Work out the finished part from the listing and answer in its coordinate system (mm). A direction names the side the tool comes from. Round coordinates to 2 decimals unless told otherwise and drop trailing zeros. Order: outer loops, then holes, each group sorted by start corner. A loop starts at its lowest first (then second) coordinate and runs counter-clockwise, first axis right, second up. Notation, with made-up numbers: M 41.25,2 L 50.25,2 A38 ccw 50.25,41 Z; hole C 85,66 d6. An arc over 180 degrees is marked long. Return JSON: item names as keys, results as strings.
from build123d import *

# Parameters (mm, degrees)
F0_R     = 19.7104
F0_R_2   = 17.1704
F1_DEPTH = 54.6227
F3_DEPTH = 19.7114
F5_DEPTH = 25.4


with BuildPart() as f1:
    # F0 (on Front) → F1 (new body, symmetric)
    with BuildSketch(Plane.XZ):
        Circle(F0_R)
        Circle(F0_R_2, mode=Mode.SUBTRACT)
    extrude(amount=F1_DEPTH, both=True)

    # F2 (on Top) → F3 (cut, through all)
    with BuildSketch(Plane.XY):
        with BuildLine():
            ThreePointArc((0, 52.7177), (-0.898026, 52.345726), (-1.27, 51.4477))
            Line((-1.27, 51.4477), (-1.27, -43.4721))
            ThreePointArc((-1.27, -43.4721), (-0.898026, -44.370126), (0, -44.7421))
            ThreePointArc((0, -44.7421), (0.898026, -44.370126), (1.27, -43.4721))
            Line((1.27, -43.4721), (1.27, 51.4477))
            ThreePointArc((1.27, 51.4477), (0.898026, 52.345726), (0, 52.7177))
        make_face()
    extrude(amount=F3_DEPTH, mode=Mode.SUBTRACT)

    # F4 (on Right) → F5 (cut, symmetric)
    with BuildSketch(Plane.YZ):
        with BuildLine():
            Line((-54.6227, 19.7104), (-54.6227, -19.7104))
            ThreePointArc((-54.6227, -19.7104), (-48.2727, 0), (-54.6227, 19.7104))
        make_face()
    extrude(amount=F5_DEPTH, both=True, mode=Mode.SUBTRACT)


solid = f1.part
Item 1: Which of the six approach directions +Z, -Z, +X, -X, +Y, -Y give full straight-line access (tool end or side, diameter ignored) to faces 4 (the cylindrical face through (14.692, -49.587, -9.331)), 5 (the flat face through (1.27, 3, 18))?
Output:
{"face 4": "+X, -X, -Y", "face 5": "+Z"}
Item 2: The mould has two halves that part along X. Classify faces 1 (the cylindrical face through (16.378, 1.582, 5.158)), 2 (the cylindrical face through (-19.69, -0.77, 0.87)), 3 (the flat face through (1, 54.623, 18)): pulls with the +X half, pulls with the -X half, needs draft (parallel to the pull), parting line crosses it, or undercut.
Output:
{"face 1": "undercut", "face 2": "parting line crosses it", "face 3": "needs draft"}
Item 3: Each of these flat-tipped pins is pushed along its axis until it touches: pin 1 (2 mm diameter, centred on y = 40.5, z = 12, fed in from -X); pin 2 (10 mm diameter, centred on y = -21.5, z = -1, fed in from +X); pin 3 (2 mm diameter, centred on x = -11.5, y = -2.5, fed in from -Z); pin 4 (1 mm diameter, centred on x = 15.5, y = 9.5, fed in from -Z). Where does it stop, or does it pass through?
Output:
{"pin 1": "stops at x = -16.36", "pin 2": "stops at x = 19.71", "pin 3": "stops at z = -16.68", "pin 4": "stops at z = -12.79"}
Item 4: Find section C-C (y = -12). Determine the outline of the cut face in (x, z), plus the area to 3 significant figures.
Output:
{"outline": "M -1.27,17.12 L -1.27,19.67 A19.71 ccw long 1.27,19.67 L 1.27,17.12 A17.17 cw long Z", "area": "288 mm^2"}
Item 5: Find section A-A (z = 0). Determine the outline of the cut face in (x, y).
Output:
{"outline": "M -19.71,-48.27 L -17.17,-48.27 L -17.17,54.62 L -19.71,54.62 Z; M 17.17,-48.27 L 19.71,-48.27 L 19.71,54.62 L 17.17,54.62 Z"}
Item 6: Find section B-B (x = -12.5). Determine the outline of the cut face in (y, z), plus the area to 3 significant figures.
Output:
{"outline": "M -51.91,-15.24 L 54.62,-15.24 L 54.62,-11.77 L -50.39,-11.77 A33.77 cw Z; M -51.91,15.24 A33.77 cw -50.39,11.77 L 54.62,11.77 L 54.62,15.24 Z", "area": "733 mm^2"}
Item 7: Consider line 1 along X through (y, z) = (0, 0); line 2 along Z through (x, y) = (0, 22); line 3 along X through (y, z) = (12.5, 8). Determine where each line is inside the solid, lowest interval first. Write a range as [from, to].
Output:
{"line 1": "x = [-19.71, -17.17], [17.17, 19.71]", "line 2": "z = [-19.71, -17.17]", "line 3": "x = [-18.01, -15.19], [15.19, 18.01]"}
